from build123d import *

# Parameters (mm, degrees)
SKETCH1_R               = 1.2
BOSS_EXTRUDE1_DEPTH     = 8
BOSS_EXTRUDE2_DEPTH     = 1.5
CUT_EXTRUDE1_DEPTH      = 125.252015178
CUT_EXTRUDE1_DEPTH_BACK = 125.252015178
SKETCH3_R               = 1.4
CUT_EXTRUDE2_DEPTH      = 125.252015178
SKETCH5_W               = 117.271867341
SKETCH5_H               = 6.016252737
CUT_EXTRUDE3_DEPTH      = 125.252015178


with BuildPart() as part:
    # Sketch1 → Boss-Extrude1 (new body)
    with BuildSketch(Plane.XY):
        with BuildLine():
            Line((32.794822831, -0.95), (98.794822831, -0.95))
            ThreePointArc((98.794822831, -0.95), (116.244822831, 16.5), (98.794822831, 33.95))
            Line((98.794822831, 33.95), (32.794822831, 33.95))
            ThreePointArc((32.794822831, 33.95), (15.344822831, 16.5), (32.794822831, -0.95))
        make_face()
        with Locations((82.294822831, 29)):
            Circle(SKETCH1_R, mode=Mode.SUBTRACT)
        with Locations((49.294822831, 4)):
            Circle(SKETCH1_R, mode=Mode.SUBTRACT)
        with Locations((82.294822831, 4)):
            Circle(SKETCH1_R, mode=Mode.SUBTRACT)
        with Locations((49.294822831, 29)):
            Circle(SKETCH1_R, mode=Mode.SUBTRACT)
        with BuildLine():
            ThreePointArc((86.132032133, 5.921543981), (82.294822831, 7.715951248), (78.457613529, 5.921543981))
            ThreePointArc((78.457613529, 5.921543981), (65.794822831, 0), (53.132032133, 5.921543981))
            ThreePointArc((53.132032133, 5.921543981), (49.294822831, 7.715951248), (45.457613529, 5.921543981))
            ThreePointArc((45.457613529, 5.921543981), (16.294822831, 16.5), (45.457613529, 27.078456019))
            ThreePointArc((45.457613529, 27.078456019), (49.294822831, 25.284048752), (53.132032133, 27.078456019))
            ThreePointArc((53.132032133, 27.078456019), (65.794822831, 33), (78.457613529, 27.078456019))
            ThreePointArc((78.457613529, 27.078456019), (82.294822831, 25.284048752), (86.132032133, 27.078456019))
            ThreePointArc((86.132032133, 27.078456019), (115.294822831, 16.5), (86.132032133, 5.921543981))
        make_face(mode=Mode.SUBTRACT)
    extrude(amount=BOSS_EXTRUDE1_DEPTH)

    # Sketch2 → Boss-Extrude2 (add)
    with BuildSketch(Plane.XY.offset(8)):
        with BuildLine():
            Line((30.807257811, -2), (100.782387851, -2))
            ThreePointArc((100.782387851, -2), (116.415253744, 7.634664408), (114.834700595, 25.929885261))
            Line((114.834700595, 25.929885261), (108.181498709, 34.893826024))
            ThreePointArc((108.181498709, 34.893826024), (108.122906141, 35.006681153), (108.102694429, 35.132223401))
            Line((108.102694429, 35.132223401), (108.102694429, 35.834314575))
            ThreePointArc((108.102694429, 35.834314575), (108.133142616, 35.987387948), (108.219851717, 36.117157288))
            Line((108.219851717, 36.117157288), (108.785537142, 36.682842712))
            ThreePointArc((108.785537142, 36.682842712), (108.872246242, 36.812612052), (108.902694429, 36.965685425))
            Line((108.902694429, 36.965685425), (108.902694429, 37.2))
            Line((108.902694429, 37.2), (22.686951233, 37.2))
            Line((22.686951233, 37.2), (22.686951233, 36.965685425))
            ThreePointArc((22.686951233, 36.965685425), (22.71739942, 36.812612052), (22.80410852, 36.682842712))
            Line((22.80410852, 36.682842712), (23.369793945, 36.117157288))
            ThreePointArc((23.369793945, 36.117157288), (23.456503046, 35.987387948), (23.486951233, 35.834314575))
            Line((23.486951233, 35.834314575), (23.486951233, 35.132223401))
            ThreePointArc((23.486951233, 35.132223401), (23.466739521, 35.006681153), (23.408146952, 34.893826024))
            Line((23.408146952, 34.893826024), (16.754945067, 25.929885261))
            ThreePointArc((16.754945067, 25.929885261), (15.174391918, 7.634664408), (30.807257811, -2))
        make_face()
    extrude(amount=BOSS_EXTRUDE2_DEPTH)

    # Sketch3 → Cut-Extrude1 (cut, two sides: drawn at the far end of the back side and taken through both)
    with BuildSketch(Plane(origin=(0, 0, 8), x_dir=(-1, 0, 0), z_dir=(0, 0, -1)).offset(-CUT_EXTRUDE1_DEPTH_BACK)):
        with Locations((-49.294822831, 29)):
            Circle(SKETCH3_R)
        with Locations((-49.294822831, 4)):
            Circle(SKETCH3_R)
        with Locations((-82.294822831, 4)):
            Circle(SKETCH3_R)
        with Locations((-82.294822831, 29)):
            Circle(SKETCH3_R)
    extrude(amount=CUT_EXTRUDE1_DEPTH + CUT_EXTRUDE1_DEPTH_BACK, mode=Mode.SUBTRACT)

    # Sketch4 → Cut-Extrude2 (cut, through all)
    with BuildSketch(Plane(origin=(0, 0, 8), x_dir=(-1, 0, 0), z_dir=(0, 0, -1))):
        with BuildLine():
            Line((-98.794822831, 25.284048752), (-32.794822831, 25.284048752))
            ThreePointArc((-32.794822831, 25.284048752), (-24.010774079, 16.5), (-32.794822831, 7.715951248))
            Line((-32.794822831, 7.715951248), (-98.794822831, 7.715951248))
            ThreePointArc((-98.794822831, 7.715951248), (-107.578871583, 16.5), (-98.794822831, 25.284048752))
        make_face()
    extrude(amount=-CUT_EXTRUDE2_DEPTH, mode=Mode.SUBTRACT)

    # Sketch5 → Cut-Extrude3 (cut, through all)
    with BuildSketch(Plane(origin=(0, 0, 8), x_dir=(-1, 0, 0), z_dir=(0, 0, -1))):
        with Locations((-71.069949673, -3.958126369)):
            Rectangle(SKETCH5_W, SKETCH5_H)
    extrude(amount=-CUT_EXTRUDE3_DEPTH, mode=Mode.SUBTRACT)


solid = part.part
For this review, take the finished solid that the model builds, in its own axes (mm). A direction names the side the tool comes from. Round coordinates to 2 decimals unless told otherwise and drop trailing zeros. Write each loop counter-clockwise with the first axis right and the second up, starting at its lowest first coordinate (ties: lowest second). Pieces come first, ordered by that corner, then holes. Notation, with made-up numbers: (16.5, 76) -> (23.5, 76) arc R25 ccw to (23.5, 101) -> close; hole circle Ø6 at (36, 72). An arc over 180 degrees is marked (long way). Use CSV: the item, a comma, the result in double quotes.
(1) For faces 1 (the face through (66, 33.95, 4)), 2 (the face through (24.013, 16.693, 8.74)), 3 (the face through (66, 35, 8)), list the 3-axis set-ups (+Z, -Z, +X, -X, +Y, -Y) from which the entire face can be reached by the end or side of a thin tool; tool diameter is ignored.
Computed values:
face 1,"-Z, +X, -X, +Y"
face 2,"+Z, -Z"
face 3,"-Z"
(2) Consider section C-C, the plane y = 29. Give the boundary of the cut face in (x, z), plus the area to 3 significant figures.
Computed values:
outline,"(19.03, 8) -> (20.62, 8) -> (20.62, 0) -> (22.02, 0) -> (22.02, 8) -> (43.57, 8) -> (43.57, 0) -> (47.89, 0) -> (47.89, 9.5) -> (19.03, 9.5) -> close; (50.69, 0) -> (55.02, 0) -> (55.02, 8) -> (76.57, 8) -> (76.57, 0) -> (80.89, 0) -> (80.89, 9.5) -> (50.69, 9.5) -> close; (83.69, 0) -> (88.02, 0) -> (88.02, 8) -> (109.57, 8) -> (109.57, 0) -> (110.97, 0) -> (110.97, 8) -> (112.56, 8) -> (112.56, 9.5) -> (83.69, 9.5) -> close"
area,"293 mm²"
(3) Consider section D-D, the plane y = 22. Give the boundary of the cut face in (x, z), plus the area to 3 significant figures.
Computed values:
outline,"(14.56, 8) -> (16.23, 8) -> (16.23, 0) -> (17.24, 0) -> (17.24, 8) -> (25.95, 8) -> (25.95, 9.5) -> (14.56, 9.5) -> close; (105.64, 8) -> (114.35, 8) -> (114.35, 0) -> (115.36, 0) -> (115.36, 8) -> (117.03, 8) -> (117.03, 9.5) -> (105.64, 9.5) -> close"
area,"50.2 mm²"
(4) Consider section B-B, the plane z = 1. Give the boundary of the cut face in (x, y).
Computed values:
outline,"(32.79, -0.95) -> (98.79, -0.95) arc R17.45 ccw to (98.79, 33.95) -> (32.79, 33.95) arc R17.45 ccw to start; hole (45.46, 5.92) arc R5 cw to (53.13, 5.92) arc R16.5 ccw to (78.46, 5.92) arc R5 cw to (86.13, 5.92) arc R16.5 ccw (long way) to (86.13, 27.08) arc R5 cw to (78.46, 27.08) arc R16.5 ccw to (53.13, 27.08) arc R5 cw to (45.46, 27.08) arc R16.5 ccw (long way) to start; hole circle Ø2.8 at (49.29, 4); hole circle Ø2.8 at (49.29, 29); hole circle Ø2.8 at (82.29, 4); hole circle Ø2.8 at (82.29, 29)"
(5) Consider section A-A, the plane y = 11. Give the boundary of the cut face in (x, z), plus the area to 3 significant figures.
Computed values:
outline,"(13.9, 8) -> (16.23, 8) -> (16.23, 0) -> (17.24, 0) -> (17.24, 8) -> (25.95, 8) -> (25.95, 9.5) -> (13.9, 9.5) -> close; (105.64, 8) -> (114.35, 8) -> (114.35, 0) -> (115.36, 0) -> (115.36, 8) -> (117.69, 8) -> (117.69, 9.5) -> (105.64, 9.5) -> close"
area,"52.2 mm²"
(6) Draft analysis for pull direction X (two halves, no side actions). For faces 4 (the face through (116.24, 16.12, 3.94)), 5 (the face through (77, 30, 0)), 6 (the face through (66, 0, 4)), state which applies: +X half, -X half, draft (parallel to the pull), parting line (faces both ways), or undercut.
Computed values:
face 4,"+X half"
face 5,"draft"
face 6,"undercut"
(7) To check wall thickness, follow L1, parallel to Y at x = 34, z = 8.5; L2, parallel to X at y = 2, z = 2.75; L3, parallel to X at y = 29, z = 4.5. State the ranges of each line that lie inside material, in increasing order. Write a range as [from, to].
Computed values:
L1,"[-0.95, 7.72], [25.28, 37.2]"
L2,"[23.09, 24.92], [40.67, 57.92], [73.67, 90.92], [106.67, 108.5]"
L3,"[20.62, 22.02], [43.57, 47.89], [50.69, 55.02], [76.57, 80.89], [83.69, 88.02], [109.57, 110.97]"
(8) Clearance check with flat-ended pins moving along their axes: P1, Ø1, axis at x = 37.5, y = 30.5, coming from the -Z side; P2, Ø1.5, axis at y = 7.5, z = 4.5, coming from the -X side; P3, Ø10, axis at x = 41, y = 20, coming from the -Z side; P4, Ø4, axis at y = 6.5, z = 6.5, coming from the -X side. State where each tip first meets the part, or that it passes through.
Computed values:
P1,"z = 8"
P2,"x = 17.42"
P3,"through"
P4,"x = 15.08"
